For this review, take the finished solid that the model builds, in its own axes (mm). A direction names the side the tool comes from. Give positions to 0.01 mm unless a question says otherwise; leave off trailing zeros. Write each loop counter-clockwise with the first axis right and the second up, starting at its lowest first coordinate (ties: lowest second). Pieces come first, ordered by that corner, then holes. Notation, with made-up numbers: M 10,-6 L 14,-6 A34 cw 14,24 Z; hole C 62.5,-37 d7. An arc over 180 degrees is marked long. Use one line per item in the form item = value. Start each with the question number.
Q1. Tool access review of faces 1 (the flat face through (0, 0, 2.381)), 2 (the cylindrical face through (-0.34, -1.55, 0.78)): name each direction out of +Z, -Z, +X, -X, +Y, -Y from which nothing blocks a thin tool from reaching the whole face with its end or side.
Q2. Consider section C-C on x = 1.25. Write out the cut boundary in (y, z), and give its area (3 significant figures).
Q3. Consider section B-B on y = 3. Write out the cut boundary in (x, z).
Q4. Consider section A-A on x = -2. Write out the cut boundary in (y, z), and give its area (3 significant figures).
Q5. Clearance check with flat-ended pins moving along their axes: pin 1 Ø0.6 at (x, y) = (0, 0) entering from -Z; pin 2 Ø0.6 at (x, z) = (4.5, 2) entering from +Y; pin 3 Ø0.9 at (x, z) = (4.5, 2) entering from -Y; pin 4 Ø1 at (x, z) = (4, 0.5) entering from +Y. State where each tip first meets the part, or that it passes through.
Q6. Mouldability with a two-part tool opening along X and no side actions: class faces 3 (the flat face through (0, 0, 1.588)), 4 (the cylindrical face through (-0.177, 4.564, 1.979)), 5 (the flat face through (1.5, 1.1, 1.588)) as released by +X, released by -X, zero draft, split by the parting line, or undercut.
Q7. For probe 1 along Z at (x, y) = (5.25, -3.5); probe 2 along X at (y, z) = (0.25, 1.1); probe 3 along Y at (x, z) = (2, 1.8), list the stretches that pass through material, from the lowest coordinate up. Write a range as [from, to].
```python
from build123d import *

# Parameters (mm, degrees)
F0_R     = 1.5875
F1_DEPTH = 1.5875
F2_W     = 1.190625
F2_H     = 1.190624
F3_W     = 1.5875
F3_H     = 1.5875
F6_DEPTH = 0.79375


with BuildPart() as f1:
    # F0 (on Top) → F1 (new body)
    with BuildSketch(Plane.XY):
        with Locations((-0.000785, 0)):
            Circle(F0_R)
    extrude(amount=F1_DEPTH)

    # F2 (on face) → F4 section 0
    with BuildSketch(Plane.XY.offset(1.5875)):
        with Locations((-1e-06, 0)):
            Rectangle(F2_W, F2_H)
    # F3 (on face) → F4 section 1
    with BuildSketch(Plane(origin=(0, 0, 0), x_dir=(1, 0, 0), z_dir=(0, 0, -1))):
        Rectangle(F3_W, F3_H)
    loft(mode=Mode.SUBTRACT)

    # F5 (on face) → F6 (join)
    with BuildSketch(Plane.XY.offset(1.5875)):
        with BuildLine():
            Line((-5.953125, 3.571875), (-5.953125, -3.571875))
            Line((-5.953125, -3.571875), (-1.190625, -3.571875))
            ThreePointArc((-1.190625, -3.571875), (-0.198438, -4.564063), (0.79375, -3.571875))
            Line((0.79375, -3.571875), (6.35, -3.571875))
            Line((6.35, -3.571875), (6.35, 3.571875))
            Line((6.35, 3.571875), (0.79375, 3.571875))
            ThreePointArc((0.79375, 3.571875), (-0.198437, 4.564063), (-1.190625, 3.571875))
            Line((-1.190625, 3.571875), (-5.953125, 3.571875))
        make_face()
    extrude(amount=F6_DEPTH)


solid = f1.part
```
Working result:
q1.face_1 = +Z, +X, -X, +Y, -Y
q1.face_2 = -Z
q2.outline = M -3.57,1.59 L -0.98,1.59 L -0.98,0 L 0.98,0 L 0.98,1.59 L 3.57,1.59 L 3.57,2.38 L -3.57,2.38 Z
q2.area = 8.77 mm²
q3.outline = M -5.95,1.59 L 6.35,1.59 L 6.35,2.38 L -5.95,2.38 Z
q4.outline = M -3.57,1.59 L 3.57,1.59 L 3.57,2.38 L -3.57,2.38 Z
q4.area = 5.67 mm²
q5.pin_1 = 1.59
q5.pin_2 = 3.57
q5.pin_3 = -3.57
q5.pin_4 = through
q6.face_3 = undercut
q6.face_4 = split by the parting line
q6.face_5 = zero draft
q7.probe_1 = [1.59, 2.38]
q7.probe_2 = [-1.57, -0.66], [0.66, 1.57]
q7.probe_3 = [-3.57, 3.57]
